```python
from build123d import *

# Parameters (mm, degrees)
SKETCH2_R          = 4
CUT_EXTRUDE1_DEPTH = 22.610182785
SKETCH3_R          = 1.409137036
SKETCH3_R_2        = 1.6
SKETCH3_R_3        = 1.49849824
SKETCH3_R_4        = 1.674312885
CUT_EXTRUDE2_DEPTH = 19.493242009


with BuildPart() as part:
    # Sketch1 → Revolve1 (revolve)
    with BuildSketch(Plane(origin=(0, 0, 0), x_dir=(1, 0, 0), z_dir=(0, 1, 0)), mode=Mode.PRIVATE) as revolve1_sk:
        Polygon((0, 0), (5.1, 0), (5.1, 1.5), (11, 1.5), (11, 5), (5.1, 5), (5.1, 15), (0, 15), align=None)
    revolve(revolve1_sk.sketch.rotate(Axis((0, 0, -15), (0, 0, 1)), 180), axis=Axis((0, 0, -15), (0, 0, 1)))

    # Sketch2 → Cut-Extrude1 (cut, through all)
    with BuildSketch(Plane(origin=(0, 0, -15), x_dir=(-1, 0, 0), z_dir=(0, 0, -1))):
        Circle(SKETCH2_R)
    extrude(amount=-CUT_EXTRUDE1_DEPTH, mode=Mode.SUBTRACT)

    # Sketch3 → Cut-Extrude2 (cut, through all)
    with BuildSketch(Plane(origin=(0, 0, -5), x_dir=(-1, 0, 0), z_dir=(0, 0, -1))):
        with Locations((8, 0)):
            Circle(SKETCH3_R)
        with Locations((0, -8)):
            Circle(SKETCH3_R_2)
        with Locations((-8, 0)):
            Circle(SKETCH3_R_3)
        with Locations((0, 8)):
            Circle(SKETCH3_R_4)
    extrude(amount=-CUT_EXTRUDE2_DEPTH, mode=Mode.SUBTRACT)


solid = part.part
```
Geometry: final body of the model. Coordinates: model frame, mm. A direction names the side the tool comes from. Coordinates: 2 decimals unless noted, no trailing zeros. Order: outer loops, then holes, each group sorted by start corner. A loop starts at its lowest first (then second) coordinate and runs counter-clockwise, first axis right, second up. Notation, with made-up numbers: (-30, 53) -> (23, 53) arc R31 cw to (23, 79) -> close; hole circle Ø9 at (1.25, -8.75). An arc over 180 degrees is marked (long way). Answer in a Markdown table with one row per item.
Item 1: Ray query, L1, parallel to Y at x = 0, z = -2.8; L2, parallel to Z at x = 5.75, y = -4.5; L3, parallel to X at y = 3, z = -1.75. Return the intervals inside material, ascending.
Return value:
| item | result |
|---|---|
| L1 | y = -11 to -9.6, -6.4 to -4, 4 to 6.33, 9.67 to 11 |
| L2 | z = -5 to -1.5 |
| L3 | x = -10.58 to -2.65, 2.65 to 10.58 |
Item 2: Section B-B on y = 8. Output: boundary loops of the cut face in (x, z), plus the area to 3 significant figures.
Return value:
| item | result |
|---|---|
| outline | (-7.55, -5) -> (-1.67, -5) -> (-1.67, -1.5) -> (-7.55, -1.5) -> close; (1.67, -5) -> (7.55, -5) -> (7.55, -1.5) -> (1.67, -1.5) -> close |
| area | 41.1 mm² |
Item 3: Access query for faces 1 (the cylindrical face through (0.22, 9.66, -3.27)), 2 (the cylindrical face through (-4.864, -1.532, -10.07)). Directions: +Z, -Z, +X, -X, +Y, -Y. A direction counts if a zero-diameter tool reaches every point of the face in a straight line with its end or side. Return the directions, or none.
Return value:
| item | result |
|---|---|
| face 1 | +Z, -Z |
| face 2 | -Z |
Item 4: Section C-C on z = -3.5. Output: boundary loops of the cut face in (x, y), plus the area to 3 significant figures.
Return value:
| item | result |
|---|---|
| outline | circle Ø22 at (0, 0); hole circle Ø2.82 at (-8, 0); hole circle Ø8 at (0, 0); hole circle Ø3.35 at (0, 8); hole circle Ø3.2 at (0, -8); hole circle Ø3 at (8, 0) |
| area | 300 mm² |
Item 5: Section D-D on x = 8. Output: boundary loops of the cut face in (y, z).
Return value:
| item | result |
|---|---|
| outline | (-7.55, -5) -> (-1.5, -5) -> (-1.5, -1.5) -> (-7.55, -1.5) -> close; (1.5, -5) -> (7.55, -5) -> (7.55, -1.5) -> (1.5, -1.5) -> close |
Item 6: Draft query along Y for faces 3 (the flat face through (5, 2, -1.5)), 4 (the cylindrical face through (-4.864, -1.532, -0.76)), 5 (the cylindrical face through (-7.695, -1.376, -3.274)). Return one class per face: released by +Y, released by -Y, zero draft, split by the parting line, or undercut.
Return value:
| item | result |
|---|---|
| face 3 | zero draft |
| face 4 | split by the parting line |
| face 5 | undercut |
Item 7: Section A-A on x = 0. Output: boundary loops of the cut face in (y, z).
Return value:
| item | result |
|---|---|
| outline | (-11, -5) -> (-9.6, -5) -> (-9.6, -1.5) -> (-11, -1.5) -> close; (-6.4, -5) -> (-5.1, -5) -> (-5.1, -15) -> (-4, -15) -> (-4, 0) -> (-5.1, 0) -> (-5.1, -1.5) -> (-6.4, -1.5) -> close; (4, -15) -> (5.1, -15) -> (5.1, -5) -> (6.33, -5) -> (6.33, -1.5) -> (5.1, -1.5) -> (5.1, 0) -> (4, 0) -> close; (9.67, -5) -> (11, -5) -> (11, -1.5) -> (9.67, -1.5) -> close |
Item 8: Contact query for flat-ended pins moving along their axis: P1, Ø2.5, axis at x = 8, y = 0, coming from the +Z side; P2, Ø6, axis at y = 1, z = -10, coming from the -X side; P3, Ø6, axis at x = 8, y = 5.5, coming from the +Z side; P4, Ø2, axis at x = 7, y = -6, coming from the -Z side. Output: stop coordinate, or through.
Return value:
| item | result |
|---|---|
| P1 | passes through |
| P2 | stops at x = -5.1 |
| P3 | stops at z = -1.5 |
| P4 | stops at z = -5 |
